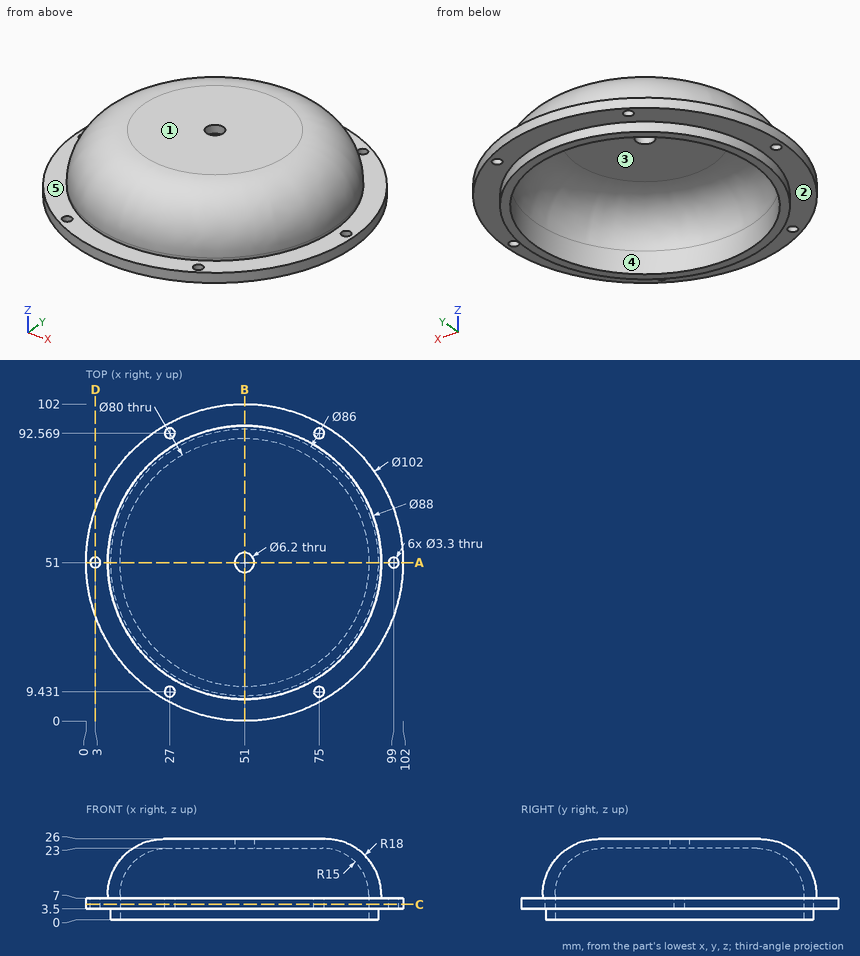
Verification items for this drawing (mm, ordinates from the low corner). A direction names the side the tool comes from. Give positions to 0.01 mm unless a question says otherwise; leave off trailing zeros. Write each loop counter-clockwise with the first axis right and the second up, starting at its lowest first coordinate (ties: lowest second). Pieces come first, ordered by that corner, then holes.
1) Thickness scan on line 1 (Z direction, x = 65, y = 70); line 2 (Y direction, x = 22, z = 6); line 3 (X direction, y = 66, z = 6.75) (1 decimal). Record the ranges inside material, lowest first.
Values follow:
line 1: z = 23 to 26
line 2: y = 9.05 to 23.45, 78.55 to 92.95
line 3: x = 2.3 to 13.9, 88.1 to 99.7
2) Set-up check for the marked faces 1 and 2: record each of +Z, -Z, +X, -X, +Y, -Y from which the full face is reachable in a straight line by a thin tool's end or side.
Values follow:
face 1: +Z, +X, -X, +Y, -Y
face 2: -Z
3) Cross-section at B-B (x = 51). Record the boundary of the cut face in (y, z), plus the area to 3 significant figures.
Values follow:
outline: (0, 3.5) - (8, 3.5) - (8, 0) - (11, 0) - (11, 8) arc R15 cw to (26, 23) - (47.9, 23) - (47.9, 26) - (25, 26) arc R18 ccw to (7, 8) - (7, 7) - (0, 7) - close; (54.1, 23) - (76, 23) arc R15 cw to (91, 8) - (91, 0) - (94, 0) - (94, 3.5) - (102, 3.5) - (102, 7) - (95, 7) - (95, 8) arc R18 ccw to (77, 26) - (54.1, 26) - close
area: 429 mm2
4) Cross-section at A-A (y = 51). Count the separate pieces of the cut face and the enclosed holes in it, plus the area to 3 significant figures.
Values follow:
separate pieces: 4
enclosed holes: 0
area: 406 mm2
5) Cross-section at C-C (z = 5). Record the boundary of the cut face in (x, y).
Values follow:
outline: circle Ø102 at (51, 51); hole circle Ø3.3 at (3, 51); hole circle Ø80 at (51, 51); hole circle Ø3.3 at (27, 9.43); hole circle Ø3.3 at (27, 92.57); hole circle Ø3.3 at (75, 9.43); hole circle Ø3.3 at (75, 92.57); hole circle Ø3.3 at (99, 51)
6) Go/stop test with flat-tipped pins: pin 1 Ø4.5 at (x, y) = (27, 9.43) entering from +Z; pin 2 Ø2.5 at (x, y) = (75, 92.57) entering from -Z; pin 3 Ø3 at (x, z) = (73.5, 15) entering from +Y; pin 4 Ø5 at (x, z) = (88.5, 13) entering from -Y. Record where each tip stops, or that it passes through.
Values follow:
pin 1: stops at z = 7
pin 2: passes through
pin 3: stops at y = 88.28
pin 4: stops at y = 25.34
7) Cross-section at D-D (x = 3). Record the boundary of the cut face in (y, z), plus the area to 3 significant figures.
Values follow:
outline: (33.77, 3.5) - (49.35, 3.5) - (49.35, 7) - (33.77, 7) - close; (52.65, 3.5) - (68.23, 3.5) - (68.23, 7) - (52.65, 7) - close
area: 109 mm2
8) Release check for a two-part mould opening along X. For the marked faces 3, 4 and 5 record: released by +X, released by -X, zero draft, split by the parting line, or undercut.
Values follow:
face 3: undercut
face 4: undercut
face 5: zero draft
